Can you work these out from the drawing? Everything is in mm from the part's minimum corner. Coordinates: 2 decimals unless noted, no trailing zeros. Loops run counter-clockwise (first coordinate to the right, second up) from the corner with the lowest first, then second, coordinate; pieces in that order, holes last. Notation, with made-up numbers: (-28, 75.5) -> (12, 75.5) arc R29 cw to (12, 103.5) -> close; hole circle Ø2 at (10.5, -20). An arc over 180 degrees is marked (long way). Use one line per item in the form item = value. Start each with the question number.
(1) I'm going to push flat-ended pins straight in: pin 1 (1 mm diameter, centred on x = 82, y = 62.5, fed in from -Z); pin 2 (1.5 mm diameter, centred on x = 3.5, z = 2, fed in from +Y); pin 3 (1.5 mm diameter, centred on x = 30.5, z = 1.5, fed in from -Y); pin 4 (0.9 mm diameter, centred on x = 59.5, z = 1, fed in from +Y). Where does each tip first touch, or does it pass through?
(2) Imagine slicing it at A-A (x = 60). List the corners of the cut face in (y, z) for me.
(3) I need wall thicknesses on line 1 (Y direction, x = 60, z = 1.75); line 2 (Y direction, x = 53, z = 2.85); line 3 (X direction, y = 6.5, z = 1.3). Which ranges of each line are inside material? Lowest first, please. Write a range as [from, to].
(4) Imagine slicing it at D-D (y = 102). List the corners of the cut face in (x, z) for me, plus the area to 3 significant figures.
(5) Imagine slicing it at B-B (z = 2.3). List the corners of the cut face in (x, y) for me.
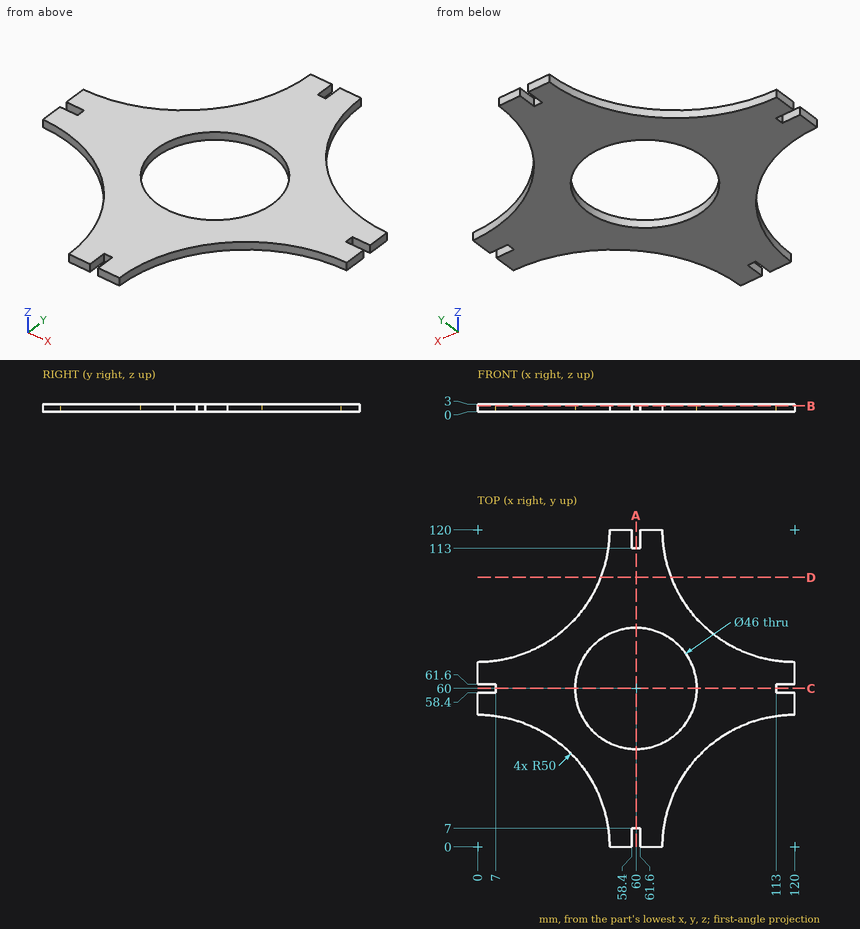
Worked out:
q1.pin_1 = through
q1.pin_2 = 70.18
q1.pin_3 = 39.03
q1.pin_4 = 113
q2.outline = (7, 0) -> (37, 0) -> (37, 3) -> (7, 3) -> close; (83, 0) -> (113, 0) -> (113, 3) -> (83, 3) -> close
q3.line_1 = [7, 37], [83, 113]
q3.line_2 = [0, 38.09], [81.91, 120]
q3.line_3 = [49.58, 58.4], [61.6, 70.42]
q4.outline = (46.65, 0) -> (73.35, 0) -> (73.35, 3) -> (46.65, 3) -> close
q4.area = 80.1 mm2
q5.outline = (0, 50) arc R50 cw to (50, 0) -> (58.4, 0) -> (58.4, 7) -> (61.6, 7) -> (61.6, 0) -> (70, 0) arc R50 cw to (120, 50) -> (120, 58.4) -> (113, 58.4) -> (113, 61.6) -> (120, 61.6) -> (120, 70) arc R50 cw to (70, 120) -> (61.6, 120) -> (61.6, 113) -> (58.4, 113) -> (58.4, 120) -> (50, 120) arc R50 cw to (0, 70) -> (0, 61.6) -> (7, 61.6) -> (7, 58.4) -> (0, 58.4) -> close; hole circle Ø46 at (60, 60)
